Part print with two shaded views. Sizes in mm from the minimum x, y, z corner. Give positions to 0.01 mm unless a question says otherwise; leave off trailing zeros. Order: outer loops, then holes, each group sorted by start corner. A loop starts at its lowest first (then second) coordinate and runs counter-clockwise, first axis right, second up. Notation, with made-up numbers: M 8,44.25 L 30,44.25 A19 ccw 30,69.25 Z; hole C -4,61.5 d2. An arc over 180 degrees is marked long. Return JSON: item names as keys, results as strings. Group by question number.
1. Wall check: probe 1 along X at (y, z) = (1.75, 70); probe 2 along Z at (x, y) = (52, 2.35); probe 3 along X at (y, z) = (0.7, 30). Give the ranges that are in metal, low to high. Write a range as [from, to].
2. Slice it at C-C on x = 85. Give the number of separate pieces and of enclosed holes in the cut face, then the cut area to 3 significant figures.
3. Slice it at B-B on x = 50. List the corners of the cut face in (y, z).
4. Slice it at A-A on z = 50. List the corners of the cut face in (x, y), then the cut area to 3 significant figures.
5. Pin check, flat tips, straight feed: pin 1 (1 mm diameter, centred on y = 0.5, z = 35.5, fed in from +X); pin 2 (1.5 mm diameter, centred on y = 2, z = 19.5, fed in from +X); pin 3 (8 mm diameter, centred on x = 15.36, z = 70, fed in from +Y). Stop position of each tip, or through.
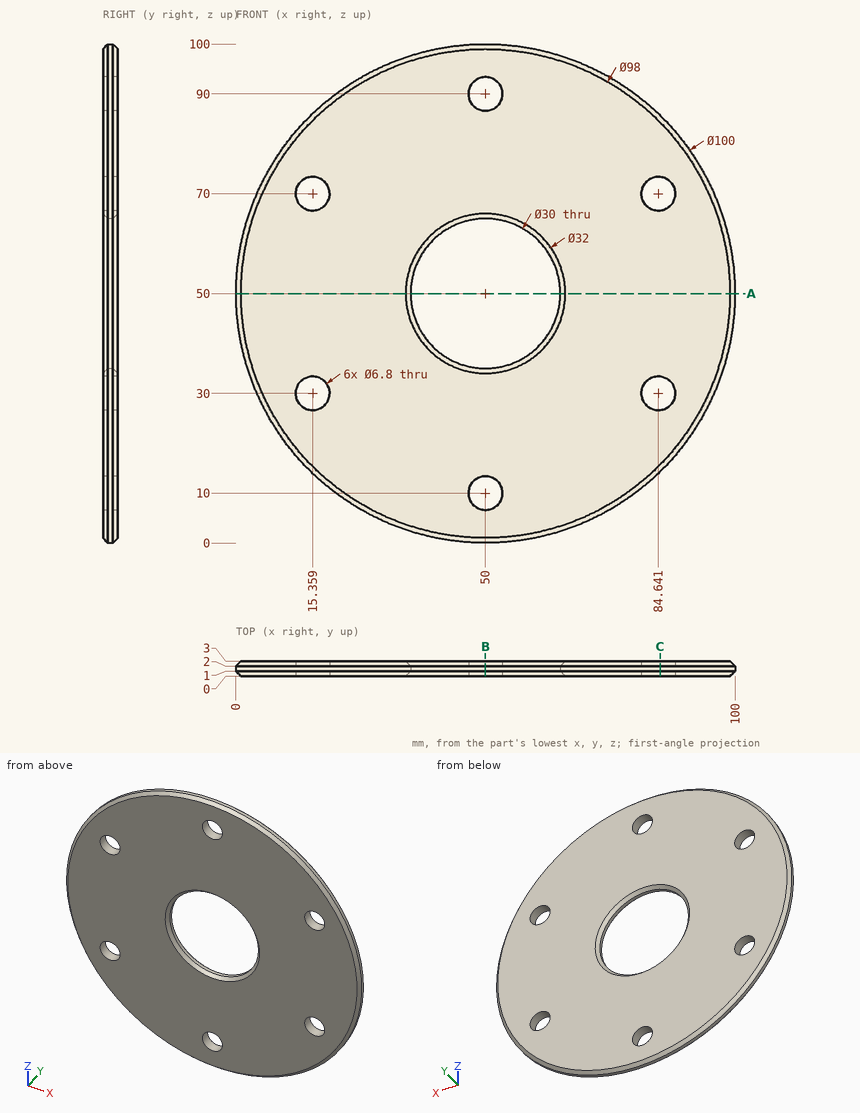
Result:
{
 "1": {"probe 1": "x = [4.17, 11.96], [18.76, 81.24], [88.04, 95.83]", "probe 2": "z = [0.39, 7.25], [12.75, 34.78], [65.22, 87.25], [92.75, 99.61]", "probe 3": "x = [4.5, 11.96], [18.76, 81.24], [88.04, 95.5]"},
 "2": {"separate pieces": "3", "enclosed holes": "0", "area": "171 mm2"},
 "3": {"outline": "M 0,1 L 1,0 L 2,0 L 3,1 L 3,6.6 L 0,6.6 Z; M 0,13.4 L 3,13.4 L 3,34 L 2,35 L 1,35 L 0,34 Z; M 0,66 L 1,65 L 2,65 L 3,66 L 3,86.6 L 0,86.6 Z; M 0,93.4 L 3,93.4 L 3,99 L 2,100 L 1,100 L 0,99 Z"},
 "4": {"outline": "M 0,1 L 1,0 L 34,0 L 35,1 L 35,2 L 34,3 L 1,3 L 0,2 Z; M 65,1 L 66,0 L 99,0 L 100,1 L 100,2 L 99,3 L 66,3 L 65,2 Z", "area": "206 mm2"},
 "5": {"pin 1": "stops at x = 97.87", "pin 2": "stops at x = 90.19", "pin 3": "stops at y = 3"}
}
